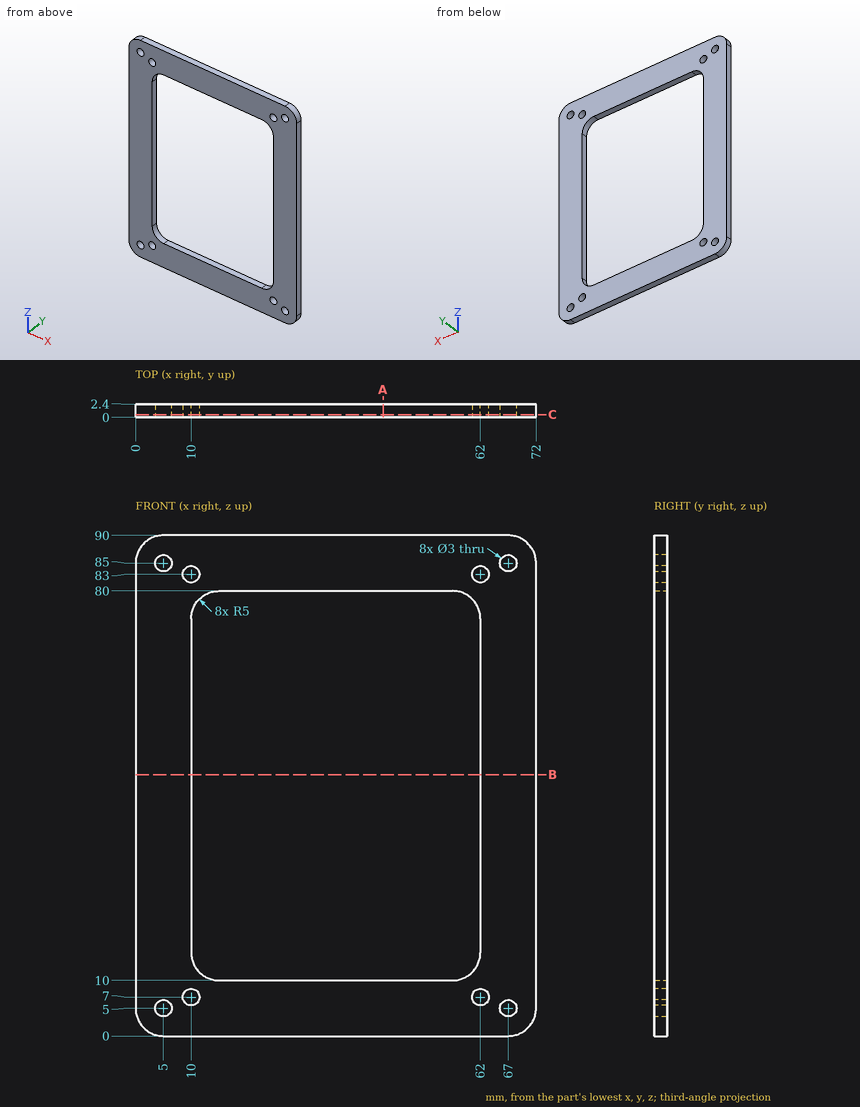
Can you work these out from the drawing? Everything is in mm from the part's minimum corner. Round coordinates to 2 decimals unless told otherwise and drop trailing zeros. Loops run counter-clockwise (first coordinate to the right, second up) from the corner with the lowest first, then second, coordinate; pieces in that order, holes last. Notation, with made-up numbers: (46.25, -24) - (55.25, -24) arc R28 ccw to (55.25, -4) - close; hole circle Ø3 at (-32, 34.25). An arc over 180 degrees is marked (long way). Answer in a Markdown table with one row per item. Add a question column.
(1) If we section it at C-C (y = 0.5): State how many separate pieces and enclosed holes the cut face has, plus the area to 3 significant figures.
(2) If we section it at A-A (x = 44.5): Please give me the cut outline in (y, z), plus the area to 3 significant figures.
(3) I need wall thicknesses on line 1 along Z through (x, y) = (5, 1.05); line 2 along X through (y, z) = (1.55, 85); line 3 along X through (y, z) = (1.3, 7). Which ranges of each line are inside material? Lowest first, please.
(4) I'm going to push flat-ended pins straight in: pin 1 (2.5 mm diameter, centred on x = 5, z = 5, fed in from +Y); pin 2 (1 mm diameter, centred on y = 1.5, z = 32.5, fed in from -X). Where does each tip first touch, or does it pass through?
(5) If we section it at B-B (z = 47): Please give me the cut outline in (x, y).
Model answer:
| question | item | result |
|---|---|---|
| 1 | separate pieces | 1 |
| 1 | enclosed holes | 9 |
| 1 | area | 2,780 mm² |
| 2 | outline | (0, 0) - (2.4, 0) - (2.4, 10) - (0, 10) - close; (0, 80) - (2.4, 80) - (2.4, 90) - (0, 90) - close |
| 2 | area | 48.0 mm² |
| 3 | line 1 | z = 0 to 3.5, 6.5 to 83.5, 86.5 to 90 |
| 3 | line 2 | x = 0 to 3.5, 6.5 to 65.5, 68.5 to 72 |
| 3 | line 3 | x = 0 to 8.5, 11.5 to 60.5, 63.5 to 72 |
| 4 | pin 1 | passes through |
| 4 | pin 2 | stops at x = 0 |
| 5 | outline | (0, 0) - (10, 0) - (10, 2.4) - (0, 2.4) - close; (62, 0) - (72, 0) - (72, 2.4) - (62, 2.4) - close |
